Autodesk Inventor part; units mm, degrees
ref_plane "4track_XY" through (0, 0, 0) normal (1, 0, 0) x (0, 0, -1)
ref_plane "4track_YZ" through (0, 0, 0) normal (0, 0, -1) x (0, 1, 0)
ref_plane "4track_ZX" through (0, 0, 0) normal (0, 1, 0) x (1, 0, 0)
sketch "Sketch_3" plane through (0, 0, 0) normal (1, 0, 0) x (0, 1, 0)
  line L0 (10.5, 13.5) -> (5.3, 13.5)
  line L1 (5.3, 13.5) -> (5.24, 13.4)
  line L2 (5.24, 13.4) -> (2.5142, 13.4)
  arc A0 (2.5142, 13.4) -> (1.8071, 13.1071) centre (2.5142, 12.4) ccw
  line L3 (1.8071, 13.1071) -> (0.2929, 11.5929)
  arc A1 (0.2929, 11.5929) -> (0, 10.8858) centre (1, 10.8858) ccw
  line L4 (0, 10.8858) -> (0, -10.8858)
  arc A2 (0, -10.8858) -> (0.2929, -11.5929) centre (1, -10.8858) ccw
  line L5 (0.2929, -11.5929) -> (1.8071, -13.1071)
  arc A3 (1.8071, -13.1071) -> (2.5142, -13.4) centre (2.5142, -12.4) ccw
  line L6 (2.5142, -13.4) -> (5.24, -13.4)
  line L7 (5.24, -13.4) -> (5.3, -13.5)
  line L8 (5.3, -13.5) -> (10.5, -13.5)
  line L9 (10.5, -13.5) -> (11, -13)
  line L10 (11, -13) -> (11, -6)
  line L11 (11, -6) -> (10.7713, -5.6188)
  arc A4 (10.7, -5.3615) -> (10.7713, -5.6188) centre (11.2, -5.3615) ccw
  line L12 (10.7, -5.3615) -> (10.7, 5.3615)
  arc A5 (10.7713, 5.6188) -> (10.7, 5.3615) centre (11.2, 5.3615) ccw
  line L13 (10.7713, 5.6188) -> (11, 6)
  line L14 (11, 6) -> (11, 13)
  line L15 (11, 13) -> (10.5, 13.5)
extrude "Extrusion1" add sketch "Sketch_3" along normal mid plane 20.6
sketch "Sketch_9" plane through (10.3, 0, 0) normal (1, 0, 0) x (0, 0, -1)
  arc A0 (-13.4, 2.5142) -> (-13.1071, 1.8071) centre (-12.4, 2.5142) ccw
  line L0 (-13.1071, 1.8071) -> (-11.5929, 0.2929)
  arc A1 (-11.5929, 0.2929) -> (-10.8858, 0) centre (-10.8858, 1) ccw
  line L1 (-10.8858, 0) -> (10.8858, 0)
  arc A2 (10.8858, 0) -> (11.5929, 0.2929) centre (10.8858, 1) ccw
  line L2 (11.5929, 0.2929) -> (13.1071, 1.8071)
  arc A3 (13.1071, 1.8071) -> (13.4, 2.5142) centre (12.4, 2.5142) ccw
  line L3 (13.4, 2.5142) -> (13.4, 9.5)
  line L4 (13.4, 9.5) -> (12.4, 10.5)
  line L5 (12.4, 10.5) -> (-12.4, 10.5)
  line L6 (-12.4, 10.5) -> (-13.4, 9.5)
  line L7 (-13.4, 9.5) -> (-13.4, 2.5142)
extrude "Extrusion2" add sketch "Sketch_9" along normal blind 6.9
sketch "Sketch_15" plane through (-10.3, 0, 0) normal (1, 0, 0) x (0, 0, -1)
  arc A0 (-13.4, 2.5142) -> (-13.1071, 1.8071) centre (-12.4, 2.5142) ccw
  line L0 (-13.1071, 1.8071) -> (-11.5929, 0.2929)
  arc A1 (-11.5929, 0.2929) -> (-10.8858, 0) centre (-10.8858, 1) ccw
  line L1 (-10.8858, 0) -> (10.8858, 0)
  arc A2 (10.8858, 0) -> (11.5929, 0.2929) centre (10.8858, 1) ccw
  line L2 (11.5929, 0.2929) -> (13.1071, 1.8071)
  arc A3 (13.1071, 1.8071) -> (13.4, 2.5142) centre (12.4, 2.5142) ccw
  line L3 (13.4, 2.5142) -> (13.4, 9.5)
  line L4 (13.4, 9.5) -> (12.4, 10.5)
  line L5 (12.4, 10.5) -> (-12.4, 10.5)
  line L6 (-12.4, 10.5) -> (-13.4, 9.5)
  line L7 (-13.4, 9.5) -> (-13.4, 2.5142)
extrude "Extrusion3" add sketch "Sketch_15" against normal blind 6.9
sketch "Sketch_40" plane through (0, 0, 0) normal (1, 0, 0) x (0, 1, 0)
  line L0 (-1.5, 6) -> (-2, 5.5)
  line L1 (-2, 5.5) -> (-2, -5.5)
  line L2 (-2, -5.5) -> (-1.5, -6)
  line L3 (-1.5, -6) -> (1.9874, -6)
  arc A0 (3.3, -5.2629) -> (1.9874, -6) centre (3.21, -6.64) ccw
  arc A1 (4.6126, -6) -> (3.3, -5.2629) centre (3.39, -6.64) ccw
  line L4 (4.6126, -6) -> (5.2, -6)
  line L5 (5.2, -6) -> (5.5, -5.7)
  line L6 (5.5, -5.7) -> (5.5, 5.7)
  line L7 (5.5, 5.7) -> (5.2, 6)
  line L8 (5.2, 6) -> (4.6126, 6)
  arc A2 (3.3, 5.2629) -> (4.6126, 6) centre (3.39, 6.64) ccw
  arc A3 (1.9874, 6) -> (3.3, 5.2629) centre (3.21, 6.64) ccw
  line L9 (1.9874, 6) -> (-1.5, 6)
extrude "Extrusion4" cut sketch "Sketch_40" along normal mid plane 34.4
sketch "Sketch5" plane through (-10.3, 11, 6) normal (0, 1, 0) x (1, 0, 0)
  point P0 (17.8, -4)
hole "Hole1" at (7.5, 11, 10) direction (0, -1, 0) diameter 2.459 depth 3.84 tip angle 120 countersink diameter 3 countersink angle 90
pattern_linear "Rectangular Pattern1" count 2 spacing 20 along (0, 0, -1) count 2 spacing 15 along (-1, 0, 0) of "Hole1"
sketch "Sketch_38" plane through (0, 0, 0) normal (0, 0, 1) x (1, 0, 0)
  line L0 (15.2, 10.5) -> (15.7, 10)
  line L1 (15.7, 10) -> (15.7, 10.5)
  line L2 (15.7, 10.5) -> (15.2, 10.5)
extrude "Extrusion5" cut sketch "Sketch_38" along normal mid plane 26.8
sketch "Sketch_39" plane through (0, 0, 0) normal (0, 0, 1) x (1, 0, 0)
  line L0 (-15.7, 10.5) -> (-15.7, 10)
  line L1 (-15.7, 10) -> (-15.2, 10.5)
  line L2 (-15.2, 10.5) -> (-15.7, 10.5)
extrude "Extrusion6" cut sketch "Sketch_39" along normal mid plane 26.8
sketch "Sketch_21" plane through (0, 0, 0) normal (0, 1, 0) x (-1, 0, 0)
  line L0 (15.7, -13.4) -> (15.7, -12.9)
  line L1 (15.7, -12.9) -> (15.2, -13.4)
  line L2 (15.2, -13.4) -> (15.7, -13.4)
extrude "Extrusion7" cut sketch "Sketch_21" along normal blind 11
sketch "Sketch_22" plane through (0, 0, 0) normal (0, 1, 0) x (-1, 0, 0)
  line L0 (-15.2, -13.4) -> (-15.7, -12.9)
  line L1 (-15.7, -12.9) -> (-15.7, -13.4)
  line L2 (-15.7, -13.4) -> (-15.2, -13.4)
extrude "Extrusion8" cut sketch "Sketch_22" along normal blind 11
sketch "Sketch_23" plane through (0, 0, 0) normal (0, 1, 0) x (-1, 0, 0)
  line L0 (-15.2, 13.4) -> (-15.7, 13.4)
  line L1 (-15.7, 13.4) -> (-15.7, 12.9)
  line L2 (-15.7, 12.9) -> (-15.2, 13.4)
extrude "Extrusion9" cut sketch "Sketch_23" along normal blind 11
sketch "Sketch_24" plane through (0, 0, 0) normal (0, 1, 0) x (-1, 0, 0)
  line L0 (15.7, 13.4) -> (15.2, 13.4)
  line L1 (15.2, 13.4) -> (15.7, 12.9)
  line L2 (15.7, 12.9) -> (15.7, 13.4)
extrude "Extrusion10" cut sketch "Sketch_24" along normal blind 11
sketch "Sketch12" plane through (17.2, 0, 0) normal (1, 0, 0) x (0, 0, -1)
  point P0 (0, 8)
hole "Hole2" at (17.2, 8, 0) direction (-1, 0, 0) diameter 2 depth 3.5
sketch "Sketch_32" plane through (0, 0, 0) normal (0, 0, 1) x (1, 0, 0)
  line L0 (-13.7, 8) -> (-17.2, 8)
  line L1 (-17.2, 8) -> (-17.2, 9)
  line L2 (-17.2, 9) -> (-13.7, 9)
  line L3 (-13.7, 9) -> (-13.7, 8)
  line L4 (-13.7, 8) -> (-17.2, 8)
revolve "Revolution1" cut sketch "Sketch_32" angle 360 about axis through (-13.7, 8, 0) along (1, 0, 0)
ref_plane "4track_XY" through (0, 0, 0) normal (1, 0, 0) x (0, 0, -1)
ref_plane "4track_YZ" through (0, 0, 0) normal (0, 0, -1) x (0, 1, 0)
ref_plane "4track_ZX" through (0, 0, 0) normal (0, 1, 0) x (1, 0, 0)
properties part number "SRS12MSS Slider" material "Steel, Alloy"
Check sheet for the modelled part. Datum: model origin and axes. Units: mm. A direction names the side the tool comes from. Coordinates: 2 decimals unless noted, no trailing zeros. Write each loop counter-clockwise with the first axis right and the second up, starting at its lowest first coordinate (ties: lowest second). Pieces come first, ordered by that corner, then holes.
Item 1: Mould release check, pull along Z, two halves, no side actions. Record for faces 1 (the face through (0, 11, 9)), 2 (the face through (-16, 6, -13.4)), 3 (the face through (-7.32, 6.57, -9.89)): released by +Z, released by -Z, zero draft, split by the parting line, or undercut.
Numbers:
face 1: zero draft
face 2: released by -Z
face 3: undercut
Item 2: Depth check by flat-ended pin: pin 1 Ø0.8 at (x, z) = (-16, 1.5) entering from +Y; pin 2 Ø2 at (x, z) = (-7.5, -10) entering from -Y; pin 3 Ø1.8 at (y, z) = (8, 0) entering from -X; pin 4 Ø2 at (x, z) = (3, -4) entering from -Y. Enter the tip coordinate at first touch or a pass-through.
Numbers:
pin 1: stops at y = 10.5
pin 2: stops at y = 0
pin 3: stops at x = -13.7
pin 4: stops at y = 5.5
Item 3: Cross-section at C-C on y = 8. Count the separate pieces of the cut face and the enclosed holes in it, then the cut area to 3 significant figures.
Numbers:
separate pieces: 1
enclosed holes: 4
area: 893 mm2
Item 4: Cross-section at B-B on z = 7. Record the boundary of the cut face in (x, y).
Numbers:
outline: (-17.2, 0) - (17.2, 0) - (17.2, 10.5) - (15.7, 10.5) - (15.7, 10) - (15.2, 10.5) - (10.3, 10.5) - (10.3, 11) - (-10.3, 11) - (-10.3, 10.5) - (-15.2, 10.5) - (-15.7, 10) - (-15.7, 10.5) - (-17.2, 10.5) - close
Item 5: Scan lines: probe 1 along Z at (x, y) = (-7.5, 9.4); probe 2 along X at (y, z) = (9.3, -10); probe 3 along Z at (x, y) = (-14.85, 8). Record each from-to range of solid material in increasing order.
Numbers:
probe 1: z = -13.5 to -11.23, -8.77 to 8.77, 11.23 to 13.5
probe 2: x = -17.2 to -8.73, -6.27 to 6.27, 8.73 to 17.2
probe 3: z = -13.4 to -1, 1 to 13.4
Item 6: Cross-section at A-A on y = 3.75. Record the boundary of the cut face in (x, z), then the cut area to 3 significant figures.
Numbers:
outline: (-17.2, -13.4) - (-15.7, -13.4) - (-15.7, -12.9) - (-15.2, -13.4) - (15.2, -13.4) - (15.7, -12.9) - (15.7, -13.4) - (17.2, -13.4) - (17.2, -5.31) - (-17.2, -5.31) - close; (-17.2, 5.31) - (17.2, 5.31) - (17.2, 13.4) - (15.7, 13.4) - (15.7, 12.9) - (15.2, 13.4) - (-15.2, 13.4) - (-15.7, 12.9) - (-15.7, 13.4) - (-17.2, 13.4) - close
area: 556 mm2
Item 7: Access from +Z, -Z, +X, -X, +Y, -Y to the whole of each face (thin tool, end or side, straight path). Record for faces 4 (the face through (-13, 10, 12.9)), 5 (the face through (-0.241, 4.075, 5.442)), 6 (the face through (16, 6, -13.4)), 7 (the face through (-13, 10, -12.9)).
Numbers:
face 4: +Z, -X, +Y
face 5: +X, -X
face 6: -Z, +X, +Y, -Y
face 7: -Z, -X, +Y
